```python
from build123d import *

# Parameters (mm, degrees)
BOSS_EXTRUDE4_DEPTH = 9.525
SKETCH6_R           = 1.27
CUT_EXTRUDE1_DEPTH  = 48.068686512


with BuildPart() as part:
    # Sketch1 → Revolve1 (revolve)
    with BuildSketch(Plane.XY, mode=Mode.PRIVATE) as revolve1_sk:
        Polygon((-28.067, 9.525), (-26.911394506, 6.35), (-23.736394506, 6.35), (-22.580789012, 9.525), (-22.072789012, 9.525), (-20.917183519, 6.35), (-17.742183519, 6.35), (-16.586578025, 9.525), (0, 9.525), (0, 0), (-28.575, 0), (-38.1, 0), (-45.1, 0), (-45.1, 4), (-38.1, 4), (-38.1, 4.254), (-28.575, 4.254), (-28.575, 9.525), align=None)
    revolve1 = revolve(revolve1_sk.sketch.rotate(Axis((-38.1, 0, 0), (1, 0, 0)), 180), axis=Axis((-38.1, 0, 0), (1, 0, 0)))

    # Sketch4 → Boss-Extrude4 (add)
    with BuildSketch(Plane.ZY.offset(28.575)):
        Polygon((0, 7.332348419), (-6.35, 3.666174209), (-6.35, -3.666174209), (0, -7.332348419), (6.35, -3.666174209), (6.35, 3.666174209), align=None)
    boss_extrude4 = extrude(amount=BOSS_EXTRUDE4_DEPTH)

    # Sketch6 → Cut-Extrude1 (cut, symmetric)
    with BuildSketch(Plane.XY):
        with Locations((-25.323894506, 0)):
            Circle(SKETCH6_R)
        with Locations((-19.329683519, 0)):
            Circle(SKETCH6_R)
    cut_extrude1 = extrude(amount=CUT_EXTRUDE1_DEPTH, both=True, mode=Mode.SUBTRACT)

    # Mirror1: Revolve1, Boss-Extrude4, Cut-Extrude1 across plane
    add(revolve1.mirror(Plane(origin=(0, 0, 0), x_dir=(0, 0, 1), z_dir=(1, 0, 0))))
    add(boss_extrude4.mirror(Plane(origin=(0, 0, 0), x_dir=(0, 0, 1), z_dir=(1, 0, 0))))
    add(cut_extrude1.mirror(Plane(origin=(0, 0, 0), x_dir=(0, 0, 1), z_dir=(1, 0, 0))), mode=Mode.SUBTRACT)


solid = part.part
```
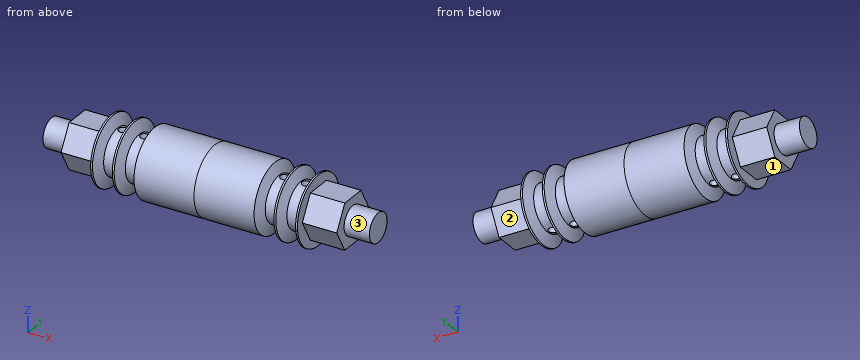
Part model, mm, in its own coordinate system. Face numbers are marked on the shaded views. A direction names the side the tool comes from. Give positions to 0.01 mm unless a question says otherwise; leave off trailing zeros. Order: outer loops, then holes, each group sorted by start corner. A loop starts at its lowest first (then second) coordinate and runs counter-clockwise, first axis right, second up. Notation, with made-up numbers: (76.25, -28.75) - (85.25, -28.75) arc R21 cw to (85.25, 3.25) - close; hole circle Ø7 at (-12, 27.25). An arc over 180 degrees is marked (long way). Use one line per item in the form item = value.
Item 1: Slice it at A-A on y = 0. Count the separate pieces of the cut face and the enclosed holes in it, and give its area (3 significant figures).
Solution:
separate_pieces = 5
enclosed_holes = 0
area = 1,200 mm2
Item 2: Slice it at B-B on x = -34.5. Give the cut face in (y, z), and give its area (3 significant figures).
Solution:
outline = (-7.33, 0) - (-3.67, -6.35) - (3.67, -6.35) - (7.33, 0) - (3.67, 6.35) - (-3.67, 6.35) - close
area = 140 mm2
Item 3: Pin check, flat tips, straight feed: pin 1 Ø1.5 at (x, z) = (-25, -2.5) entering from +Y; pin 2 Ø8 at (x, y) = (-31, -0.5) entering from +Z (3 decimals); pin 3 Ø2 at (x, y) = (34.5, -1) entering from +Z; pin 4 Ø1 at (x, y) = (34.5, 1) entering from -Z. Stop position of each tip, or through.
Solution:
pin_1 = 6.1
pin_2 = 9.525
pin_3 = 6.35
pin_4 = -6.35
Item 4: Which spindle directions (+Z, -Z, +X, -X, +Y, -Y) get a long thin tool onto all of the face, cutting with end or side? Do the marked faces 1, 2 and 3. Say none if no direction does.
Solution:
face_1 = -Z, -X, +Y, -Y
face_2 = -Z, +X, +Y
face_3 = +X
Item 5: Probe probe 1 along X at (y, z) = (0, -2.75); probe 2 along X at (y, z) = (4.25, -5.5) (3 decimals); probe 3 along Z at (x, y) = (-32.5, -1.5). List the from-to ranges inside material, lowest first. Write a range as from..to.
Solution:
probe_1 = -45.1..-26.59, -24.05..-20.6, -18.06..18.06, 20.6..24.05, 26.59..45.1
probe_2 = -28.575..-27.13, -23.518..-21.136, -17.524..17.524, 21.136..23.518, 27.13..28.575
probe_3 = -6.35..6.35
Item 6: Slice it at D-D on x = -14. Give the cut face in (y, z) (3 decimals).
Solution:
outline = circle Ø19.05 at (0, 0)
